Check sheet for the modelled part. Datum: model origin and axes. Units: mm. A direction names the side the tool comes from. Coordinates: 2 decimals unless noted, no trailing zeros. Order: outer loops, then holes, each group sorted by start corner. A loop starts at its lowest first (then second) coordinate and runs counter-clockwise, first axis right, second up. Notation, with made-up numbers: (9, 10) -> (27, 10) arc R9 ccw to (27, 24) -> close; hole circle Ø1 at (-37, 74.5). An arc over 180 degrees is marked (long way). Put each result on its own line as item: value. Start each with the question number.
Autodesk Inventor part; units mm, degrees
ref_plane "YZ Plane" through (0, 0, 0) normal (1, 0, 0) x (0, 1, 0)
ref_plane "XZ Plane" through (0, 0, 0) normal (0, 1, 0) x (-1, 0, 0)
ref_plane "XY Plane" through (0, 0, 0) normal (0, 0, 1) x (1, 0, 0)
sketch "Szkic1" plane through (0, 0, 0) normal (0, 1, 0) x (-1, 0, 0)
  line L0 (-60, 42.2624) -> (60, 42.2624)
  line L1 (60, 42.2624) -> (60, -41.7376)
  line L2 (60, -41.7376) -> (-60, -41.7376)
  line L3 (-60, -41.7376) -> (-60, 42.2624)
  line L4 (-34.5, 26.7624) -> (34.5, 26.7624)
  line L5 (34.5, 26.7624) -> (34.5, -26.2376)
  line L6 (34.5, -26.2376) -> (-34.5, -26.2376)
  line L7 (-34.5, -26.2376) -> (-34.5, 26.7624)
  line L8 (39.5, 37.2624) -> (55, 37.2624)
  line L9 (55, 37.2624) -> (55, -36.7376)
  line L10 (55, -36.7376) -> (39.5, -36.7376)
  line L11 (39.5, -36.7376) -> (39.5, 37.2624)
  line L12 (39.5, 37.2624) -> (55, -36.7376) construction
  line L13 (55, 37.2624) -> (39.5, -36.7376) construction
  line L14 (-39.5, 37.2624) -> (-55, 37.2624)
  line L15 (-55, 37.2624) -> (-55, -36.7376)
  line L16 (-55, -36.7376) -> (-39.5, -36.7376)
  line L17 (-39.5, -36.7376) -> (-39.5, 37.2624)
  line L18 (-39.5, 37.2624) -> (-55, -36.7376) construction
  line L19 (-55, 37.2624) -> (-39.5, -36.7376) construction
  circle A0 centre (19.5, -23.2376) radius 1.3
  line L20 (0, 0) -> (11.1545, 0)
  circle A1 centre (20.5, 23.7624) radius 1.3
  circle A2 centre (-31.5, 18.7624) radius 1.3
  circle A3 centre (20.5, 23.7624) radius 1.3
  circle A4 centre (19.5, -23.2376) radius 1.3
  circle A5 centre (-31.5, 18.7624) radius 1.3
  point P0 (47.25, 0.2624)
  dimension "d0" = 120
  dimension "d1" = 84
  dimension "d4" = 69
  dimension "d5" = 53
  dimension "d8" = 5
  dimension "d9" = 5
  dimension "d13" = 2.6
  dimension "d14" = 3
  dimension "d15" = 15
  dimension "d16" = 15.5
  dimension "d17" = 15.5
  dimension "d18" = 25.5
  dimension "d19" = 5
  dimension "d20" = 5
  dimension "d23" = 2.6
  dimension "d24" = 3
  dimension "d25" = 14
  dimension "d28" = 2.6
extrude "Wyciągnięcie proste1" add sketch "Szkic1" along normal blind 2 contours L0 L1 L2 L3 | L4 L5 L6 L7 | A0 | A1 | A2
sketch "Szkic3" plane through (0, 0, 0) normal (0, -1, 0) x (1, 0, 0)
  circle A0 centre (-20.5, 23.7624) radius 1.3
  circle A1 centre (31.5, 18.7624) radius 1.3
  circle A2 centre (-19.5, -23.2376) radius 1.3
  circle A3 centre (-19.5, -23.2376) radius 1.3
  circle A4 centre (-20.5, 25.0124) radius 1.3
  line L0 (31.5, 18.7624) -> (31.5, 19.7624)
  circle A5 centre (31.5, 19.7624) radius 1.3
  point P0 (0, 0)
  dimension "d31" = 2.6
  dimension "d32" = 48.25
  dimension "d36" = 1
extrude "Wyciągnięcie proste2" add sketch "Szkic3" against normal blind 5 contours A4 A0 | A0 A4 | A5 A1 | A1 A5 | A2 picked at (-20.4486, 24.1655) picked at (-20.5582, 25.8863) picked at (31.399, 19.5171) picked at (31.6684, 20.3785)
sketch "Szkic4" plane through (0, 0, 0) normal (0, -1, 0) x (1, 0, 0)
  arc A0 (-21.6399, 24.3874) -> (-19.3601, 24.3874) centre (-20.5, 23.7624) ccw
  circle A1 centre (-20.5, 23.7624) radius 1.3
  arc A2 (30.3, 19.2624) -> (32.7, 19.2624) centre (31.5, 18.7624) ccw
  circle A3 centre (31.5, 18.7624) radius 1.3
  point P0 (0, 0)
  point P1 (32.7, 19.2624)
extrude "Wyciągnięcie proste3" add sketch "Szkic4" against normal blind 2
sketch "Szkic5" plane through (-60, 0, 42.2624) normal (0, 0, 1) x (1, 0, 0)
  line L0 (0, 0) -> (0, 2)
  line L1 (5, 0) -> (20.5, 0)
  line L2 (0, 0) -> (20.5, 0)
  line L3 (5, 2) -> (20.5, 2)
  line L4 (20.5, 0) -> (20.5, 2)
  line L5 (20.5, 2) -> (0, 2)
  line L6 (0, 2) -> (0, 0)
  point P0 (60, 0)
extrude "Wyciągnięcie proste4" cut sketch "Szkic5" against normal up to surface (84 mm away)
properties part number "gora"
1) Scan lines: line 1 along X through (y, z) = (0.35, 36); line 2 along Y through (x, z) = (-24.5, -17); line 3 along Z through (x, y) = (-20.5, 4.05). Record each from-to range of solid material in increasing order. Write a range as [from, to].
2) Access from +Z, -Z, +X, -X, +Y, -Y to the whole of each face (thin tool, end or side, straight path). Record for faces 4 (the flat face through (-20, 5, -23)), 5 (the cylindrical face through (30.2, 3.5, 19.8)), 6 (the flat face through (39.5, 1, 0)).
3) Mould release check, pull along X, two halves, no side actions. Record for faces 1 (the cylindrical face through (-20.53, 3.48, -24.03)), 2 (the flat face through (-39.5, 1, 1)), 3 (the flat face through (47, 1, 37.262)): +X half, -X half, draft (parallel to the pull), parting line (faces both ways), or undercut.
4) Sectioned sample at C-C (x = 31.5). Record the boundary of the cut face in (y, z).
5) Gauge pin test, flat ends, axial feed: pin 1 (6 mm diameter, centred on x = 45, z = -15.5, fed in from +Y); pin 2 (12 mm diameter, centred on x = -1.5, z = -11, fed in from +Y); pin 3 (1.5 mm diameter, centred on x = -3, z = 16, fed in from -Y). Record the tip position at first contact, or that the pin passes through.
6) Sectioned sample at D-D (y = 3.25). Record the boundary of the cut face in (x, z), plus the area to 3 significant figures.
7) Sectioned sample at B-B (x = 51.5). Record the boundary of the cut face in (y, z).
8) Sectioned sample at A-A (z = 35). Record the boundary of the cut face in (x, y), plus the area to 3 significant figures.
Entries:
1. line 1: x = [-39.5, 39.5], [55, 60]
1. line 2: y = [0, 2]
1. line 3: z = [-24.07, -22.41], [23.71, 26.31]
2. face 4: +Z, -Z, +X, -X, +Y
2. face 5: +Y
2. face 6: +Y, -Y
3. face 1: parting line
3. face 2: -X half
3. face 3: undercut
4. outline: (0, -41.74) -> (2, -41.74) -> (2, 18.46) -> (5, 18.46) -> (5, 21.06) -> (2, 21.06) -> (2, 42.26) -> (0, 42.26) -> close
5. pin 1: passes through
5. pin 2: stops at y = 2
5. pin 3: stops at y = 0
6. outline: circle Ø2.6 at (-20.5, 25.01); circle Ø2.6 at (-19.5, -23.24); circle Ø2.6 at (31.5, 19.76)
6. area: 15.9 mm2
7. outline: (0, -41.74) -> (2, -41.74) -> (2, -36.74) -> (0, -36.74) -> close; (0, 37.26) -> (2, 37.26) -> (2, 42.26) -> (0, 42.26) -> close
8. outline: (-39.5, 0) -> (39.5, 0) -> (39.5, 2) -> (-39.5, 2) -> close; (55, 0) -> (60, 0) -> (60, 2) -> (55, 2) -> close
8. area: 168 mm2
